```python
from build123d import *

# Parameters (mm, degrees)
SKETCH1_R           = 7.5
SKETCH1_R_2         = 4.9
SKETCH1_R_3         = 2.4
SKETCH1_W           = 188
SKETCH1_H           = 9
BOSS_EXTRUDE1_DEPTH = 2
CUT_EXTRUDE1_DEPTH  = 208.645129969


with BuildPart() as part:
    # Sketch1 → Boss-Extrude1 (new body)
    # profile 1 of 3: a face of its own
    with BuildSketch(Plane.XY):
        Circle(SKETCH1_R)
        Circle(SKETCH1_R_2, mode=Mode.SUBTRACT)
    # profile 2 of 3: a face of its own
    with BuildSketch(Plane.XY):
        with Locations((200, 0)):
            Circle(SKETCH1_R)
        with Locations((200, 0)):
            Circle(SKETCH1_R_3, mode=Mode.SUBTRACT)
    # profile 3 of 3: a face of its own
    with BuildSketch(Plane.XY):
        with Locations((100, 0)):
            Rectangle(SKETCH1_W, SKETCH1_H)
    extrude(amount=BOSS_EXTRUDE1_DEPTH)

    # Sketch2 → Cut-Extrude1 (cut, through all)
    with BuildSketch(Plane.XY.offset(2)):
        with BuildLine():
            Line((75, 2.5), (125, 2.5))
            ThreePointArc((125, 2.5), (127.5, 0), (125, -2.5))
            Line((125, -2.5), (75, -2.5))
            ThreePointArc((75, -2.5), (72.5, 0), (75, 2.5))
        make_face()
        with BuildLine():
            Line((135, 2.5), (185, 2.5))
            ThreePointArc((185, 2.5), (187.5, 0), (185, -2.5))
            Line((185, -2.5), (135, -2.5))
            ThreePointArc((135, -2.5), (132.5, 0), (135, 2.5))
        make_face()
        with BuildLine():
            Line((15, 2.5), (65, 2.5))
            ThreePointArc((65, 2.5), (67.5, 0), (65, -2.5))
            Line((65, -2.5), (15, -2.5))
            ThreePointArc((15, -2.5), (12.5, 0), (15, 2.5))
        make_face()
    extrude(amount=-CUT_EXTRUDE1_DEPTH, mode=Mode.SUBTRACT)


solid = part.part
```
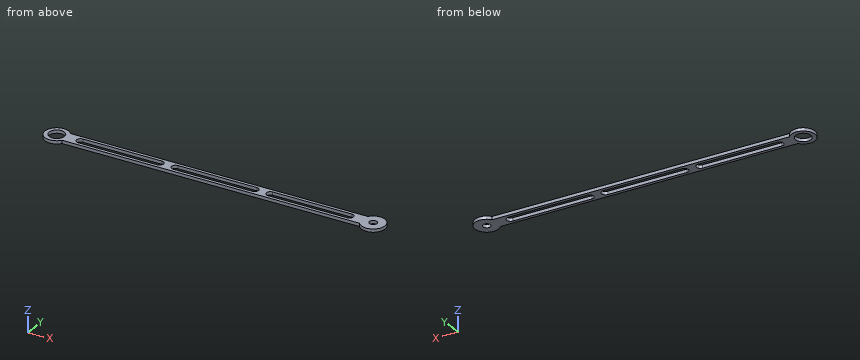
Geometry: final body of the model. Coordinates: model frame, mm. Give positions to 0.01 mm unless a question says otherwise; leave off trailing zeros. Order: outer loops, then holes, each group sorted by start corner. A loop starts at its lowest first (then second) coordinate and runs counter-clockwise, first axis right, second up. Notation, with made-up numbers: (67, 78.5) -> (84, 78.5) arc R36 cw to (84, 114.5) -> close; hole circle Ø10 at (62, 51.5). An arc over 180 degrees is marked (long way). Write each question's results on one line, items separated by ' | '. Start each with the question number.
1) Line query: line 1 (X direction, y = -0.25, z = 1.9); line 2 (Y direction, x = 147, z = 0.75); line 3 (Y direction, x = 200, z = 1.15). Output: solid intervals per line, ascending. Write a range as from..to.
2) Section A-A (x = 152.5). Return loops of the section in (y, z), then the cut area to 3 significant figures.
3) Section D-D (x = 130). Return loops of the section in (y, z).
4) Section C-C (x = 0). Return loops of the section in (y, z), then the cut area to 3 significant figures.
5) Section B-B (z = 1.3). Return loops of the section in (x, y), then the cut area to 3 significant figures.
6) First-contact query: pin 1 (1 mm diameter, centred on y = 2.5, z = 0.5, fed in from -X); pin 2 (2 mm diameter, centred on x = 137.5, y = 6, fed in from -Z); pin 3 (1 mm diameter, centred on x = 167, z = 0.5, fed in from +Y); pin 4 (1 mm diameter, centred on x = 158.5, z = 1.5, fed in from -Y). Flat tips, straight axial feed; report the tip coordinate or a pass-through.
Calculated:
1) line 1: -7.5..-4.89, 4.89..12.51, 67.49..72.51, 127.49..132.51, 187.49..197.61, 202.39..207.5 | line 2: -4.5..-2.5, 2.5..4.5 | line 3: -7.5..-2.4, 2.4..7.5
2) outline: (-4.5, 0) -> (-2.5, 0) -> (-2.5, 2) -> (-4.5, 2) -> close; (2.5, 0) -> (4.5, 0) -> (4.5, 2) -> (2.5, 2) -> close | area: 8.00 mm2
3) outline: (-4.5, 0) -> (4.5, 0) -> (4.5, 2) -> (-4.5, 2) -> close
4) outline: (-7.5, 0) -> (-4.9, 0) -> (-4.9, 2) -> (-7.5, 2) -> close; (4.9, 0) -> (7.5, 0) -> (7.5, 2) -> (4.9, 2) -> close | area: 10.4 mm2
5) outline: (6, -4.5) -> (194, -4.5) arc R7.5 ccw (long way) to (194, 4.5) -> (6, 4.5) arc R7.5 ccw (long way) to start; hole circle Ø9.8 at (0, 0); hole (15, -2.5) -> (65, -2.5) arc R2.5 ccw to (65, 2.5) -> (15, 2.5) arc R2.5 ccw to start; hole (75, -2.5) -> (125, -2.5) arc R2.5 ccw to (125, 2.5) -> (75, 2.5) arc R2.5 ccw to start; hole (135, -2.5) -> (185, -2.5) arc R2.5 ccw to (185, 2.5) -> (135, 2.5) arc R2.5 ccw to start; hole circle Ø4.8 at (200, 0) | area: 1,120 mm2
6) pin 1: x = -7.23 | pin 2: through | pin 3: y = 4.5 | pin 4: y = -4.5
